```python
from build123d import *

# Parameters (mm, degrees)
BOSS_EXTRUDE1_DEPTH = 9.3
CUT_EXTRUDE1_DEPTH  = 42.511134509
CUT_EXTRUDE2_DEPTH  = 42.511134509
HOLE1_D             = 3.5
HOLE2_D             = 3.5
FILLET1_R           = 0.6
FILLET2_R           = 5


with BuildPart() as part:
    # Sketch1 → Boss-Extrude1 (new body)
    with BuildSketch(Plane(origin=(-27.480838388, 0, 0), x_dir=(0, 0, -1), z_dir=(1, 0, 0))):
        with BuildLine():
            Line((81.963336874, -40.96995038), (76.413336874, -52.210980091))
            ThreePointArc((76.413336874, -52.210980091), (78.229167535, -57.568475682), (83.586663126, -55.752645021))
            Line((83.586663126, -55.752645021), (89.136663126, -44.51161531))
            ThreePointArc((89.136663126, -44.51161531), (87.320832465, -39.154119719), (81.963336874, -40.96995038))
        make_face()
    extrude(amount=-BOSS_EXTRUDE1_DEPTH)

    # Sketch2 → Cut-Extrude1 (cut, through all)
    with BuildSketch(Plane(origin=(0, -44.107651135, -89.336111151), x_dir=(-1, 0, 0), z_dir=(0, -0.4427081162196108, -0.8966657815670697))):
        Polygon((31.280838388, 3.94822391), (31.280838388, -4.049700743), (36.780838388, -7.974283766), (36.780838388, 3.94822391), align=None)
    extrude(amount=-CUT_EXTRUDE1_DEPTH, mode=Mode.SUBTRACT)

    # Sketch3 → Cut-Extrude2 (cut, through all)
    with BuildSketch(Plane(origin=(0, -44.107651135, -89.336111151), x_dir=(-1, 0, 0), z_dir=(0, -0.4427081162196108, -0.8966657815670697))):
        Polygon((32.980838388, -17.88847919), (32.980838388, -8.986994848), (27.480838388, -4.88847919), (27.480838388, -17.88847919), align=None)
    extrude(amount=-CUT_EXTRUDE2_DEPTH, mode=Mode.SUBTRACT)

    # Hole1 (through all)
    with Locations(Plane.ZY.offset(36.780838388)):
        with Locations((-80, -53.981812556)):
            Hole(HOLE1_D / 2)

    # Hole2 (through all)
    with Locations(Plane.ZY.offset(31.280838388)):
        with Locations((-85.55, -42.740782845)):
            Hole(HOLE2_D / 2)

    # Fillet1
    fillet1_edges = [part.edges().sort_by_distance(p)[0] for p in [
        (-31.280838388, -45.968046752, -83.956612638),
        (-32.980838388, -50.395149429, -81.770832465),
    ]]
    fillet(fillet1_edges, radius=FILLET1_R)

    # Fillet2
    fillet2_edges = [part.edges().sort_by_distance(p)[0] for p in [
        (-36.780838388, -49.487086055, -82.21916788),
        (-27.480838388, -46.720150684, -83.585278611),
    ]]
    fillet(fillet2_edges, radius=FILLET2_R)


solid = part.part
```
Verification items for the finished model (mm, model axes). A direction names the side the tool comes from. Give positions to 0.01 mm unless a question says otherwise; leave off trailing zeros. Order: outer loops, then holes, each group sorted by start corner. A loop starts at its lowest first (then second) coordinate and runs counter-clockwise, first axis right, second up. Notation, with made-up numbers: M 11,-36 L 49,-36 A28 cw 49,-1 Z; hole C 89.5,6 d3. An arc over 180 degrees is marked long. Answer in a Markdown table with one row per item. Add a question column.
Item 1: Section check B-B, the plane x = -34.25. Enter the section's corners in (y, z).
Item 2: Mould release check, pull along Z, two halves, no side actions. Record for faces 1 (the cylindrical face through (-31.35, -45.92, -83.92)), 2 (the cylindrical face through (-29.35, -44.45, -85.17)), 3 (the flat face through (-31.281, -43.2, -87.4)): released by +Z, released by -Z, zero draft, split by the parting line, or undercut.
Item 3: Tool access check on faces 4 (the flat face through (-32.066, -50.211, -86.323)), 5 (the flat face through (-32.981, -53, -82)). Record the directions out of +Z, -Z, +X, -X, +Y, -Y that give a thin tool (end or side, any length) a straight path to the whole face; none if there is none.
Item 4: Scan lines: probe 1 along X at (y, z) = (-42.5, -83); probe 2 along Y at (x, z) = (-35.6, -80); probe 3 along Y at (x, z) = (-29.7, -85.55). Record each from-to range of solid material in increasing order. Write a range as from..to.
Item 5: Section check D-D, the plane x = -32.5. Enter the section's corners in (y, z), and give its area (3 significant figures).
Item 6: Section check A-A, the plane y = -54.5. Enter the section's corners in (x, z), and give its area (3 significant figures).
Item 7: Gauge pin test, flat ends, axial feed: pin 1 (5 mm diameter, centred on y = -44.5, z = -87, fed in from -X); pin 2 (4.5 mm diameter, centred on y = -53.5, z = -82.5, fed in from +X); pin 3 (4 mm diameter, centred on x = -29, z = -78.5, fed in from +Y); pin 4 (6 mm diameter, centred on y = -49, z = -87.5, fed in from +X). Record the tip position at first contact, or that the pin passes through.
Item 8: Section check C-C, the plane x = -30.5. Enter the section's corners in (y, z).
Filled sheet:
| question | item | result |
|---|---|---|
| 1 | outline | M -55.75,-83.59 L -49.64,-86.61 L -46.1,-79.43 L -52.21,-76.41 A4 ccw Z; hole C -53.98,-80 d3.5 |
| 2 | face 1 | released by -Z |
| 2 | face 2 | undercut |
| 2 | face 3 | zero draft |
| 3 | face 4 | -Z, +X, -X, -Y |
| 3 | face 5 | +Z, +X, -Y |
| 4 | probe 1 | x = -31.28..-27.48 |
| 4 | probe 2 | y = -57.98..-55.73, -52.23..-47.66 |
| 4 | probe 3 | y = -49.53..-44.49, -40.99..-38.74 |
| 5 | outline | M -51.84,-85.52 L -48.52,-87.16 L -44.98,-79.98 L -48.3,-78.34 Z |
| 5 | area | 29.7 mm^2 |
| 6 | outline | M -36.78,-84.21 L -32.98,-84.21 L -32.98,-81.67 L -36.78,-81.67 Z; M -36.78,-78.33 L -32.98,-78.33 L -32.98,-76.03 L -36.78,-76.03 Z |
| 6 | area | 18.3 mm^2 |
| 7 | pin 1 | stops at x = -31.3 |
| 7 | pin 2 | stops at x = -32.97 |
| 7 | pin 3 | stops at y = -43.93 |
| 7 | pin 4 | stops at x = -27.48 |
| 8 | outline | M -50.51,-86.18 L -44.51,-89.14 A4 ccw -40.97,-81.96 L -46.97,-79 Z; hole C -42.74,-85.55 d3.5 |
